Autodesk Inventor part; units mm, degrees
ref_plane "YZ Plane" through (0, 0, 0) normal (1, 0, 0) x (0, 1, 0)
ref_plane "XZ Plane" through (0, 0, 0) normal (0, 1, 0) x (-1, 0, 0)
ref_plane "XY Plane" through (0, 0, 0) normal (0, 0, 1) x (1, 0, 0)
sketch "Sketch1" plane through (0, 0, 0) normal (0, 0, 1) x (1, 0, 0)
  circle A0 centre (0, 0) radius 9.1281
  dimension "d0" = 18.2563
  dimension "d1" = 0
extrude "Extrusion1" add sketch "Sketch1" against normal blind 11.1125
sketch "Sketch2" plane through (0, 0, 0) normal (0, 0, 1) x (1, 0, 0)
  circle A0 centre (0, 0) radius 10.3188
  dimension "d15" = 20.6375
extrude "Extrusion2" add sketch "Sketch2" along normal blind 9.525
hole "Hole1" at (0, 0, 9.525) direction (0, 0, -1) diameter 13.0969 end through all
thread "Thread2"
sketch "Sketch3" plane through (0, 0, 9.525) normal (0, 0, 1) x (1, 0, 0)
  line L0 (0, -7.6975) -> (0, 10.1618) construction
  line L1 (0, 11.43) -> (1.1906, 11.43)
  line L2 (1.1906, 11.43) -> (1.1906, -11.43)
  line L3 (1.1906, -11.43) -> (0, -11.43)
  line L4 (0, 11.43) -> (-1.1906, 11.43)
  line L5 (-1.1906, 11.43) -> (-1.1906, -11.43)
  line L6 (-1.1906, -11.43) -> (0, -11.43)
  point P0 (0, 0)
  dimension "d22" = 1.1906
  dimension "d23" = 11.43
  dimension "d24" = 11.43
extrude "Extrusion3" cut sketch "Sketch3" against normal blind 3.175
properties part number "VS-005(COLLAR)" material "Steel, Carbon"
Geometry check sheet. Reference: the model listing, model coordinates, mm. A direction names the side the tool comes from. Coordinates: 2 decimals unless noted, no trailing zeros. Loops run counter-clockwise (first coordinate to the right, second up) from the corner with the lowest first, then second, coordinate; pieces in that order, holes last.
Item 1: Access from +Z, -Z, +X, -X, +Y, -Y to the whole of each face (thin tool, end or side, straight path). Record for faces 4 (the face through (6, -4, -11.112)), 5 (the face through (2.2, -9.1, 0)), 6 (the face through (-1.191, -8, 8)).
Item 2: Sectioned sample at A-A, the plane x = 0. Record the boundary of the cut face in (y, z), then the cut area to 3 significant figures.
Item 3: Sectioned sample at B-B, the plane y = 0. Record the boundary of the cut face in (x, z) (1 decimal), then the cut area to 3 significant figures.
Item 4: Go/stop test with flat-tipped pins: pin 1 Ø1 at (y, z) = (4.5, -8.5) entering from +X (3 decimals); pin 2 Ø1.2 at (x, y) = (0.5, 8) entering from +Z; pin 3 Ø1 at (y, z) = (-1.5, -5.5) entering from +X. Record where each tip stops, or that it passes through.
Item 5: Thickness scan on line 1 (X direction, y = 0, z = 3.5); line 2 (Y direction, x = 0, z = -0.75). Record the ranges inside material, lowest first.
Item 6: Sectioned sample at C-C, the plane z = -6.75. Record the boundary of the cut face in (x, y), then the cut area to 3 significant figures.
Item 7: Release check for a two-part mould opening along X. For faces 1 (the face through (7, 0, 9.525)), 2 (the face through (-1.191, 8, 8)), 3 (the face through (-7.61, -6.97, 4.7)) record: released by +X, released by -X, zero draft, split by the parting line, or undercut.
Check result:
1. face 4: -Z, +X, -X, +Y, -Y
1. face 5: -Z
1. face 6: +Z, +Y, -Y
2. outline: (-10.32, 0) - (-9.13, 0) - (-9.13, -11.11) - (-6.55, -11.11) - (-6.55, 6.35) - (-10.32, 6.35) - close; (6.55, -11.11) - (9.13, -11.11) - (9.13, 0) - (10.32, 0) - (10.32, 6.35) - (6.55, 6.35) - close
2. area: 105 mm2
3. outline: (-10.3, 0) - (-9.1, 0) - (-9.1, -11.1) - (-6.5, -11.1) - (-6.5, 9.5) - (-10.3, 9.5) - close; (6.5, -11.1) - (9.1, -11.1) - (9.1, 0) - (10.3, 0) - (10.3, 9.5) - (6.5, 9.5) - close
3. area: 129 mm2
4. pin 1: stops at x = 8.205
4. pin 2: stops at z = 6.35
4. pin 3: stops at x = 9.07
5. line 1: x = -10.32 to -6.55, 6.55 to 10.32
5. line 2: y = -9.13 to -6.55, 6.55 to 9.13
6. outline: circle Ø18.26 at (0, 0); hole circle Ø13.1 at (0, 0)
6. area: 127 mm2
7. face 1: zero draft
7. face 2: undercut
7. face 3: split by the parting line
